Drawing for the job (mm, zero at the part's lowest x, y, z). Give positions to 0.01 mm unless a question says otherwise; leave off trailing zeros. Order: outer loops, then holes, each group sorted by start corner. A loop starts at its lowest first (then second) coordinate and runs counter-clockwise, first axis right, second up. Notation, with made-up numbers: M 24.25,-18 L 78.25,-18 A14 ccw 78.25,-14 Z; hole C 74,28.25 d2. An arc over 180 degrees is marked long. One line per item, written item: value.
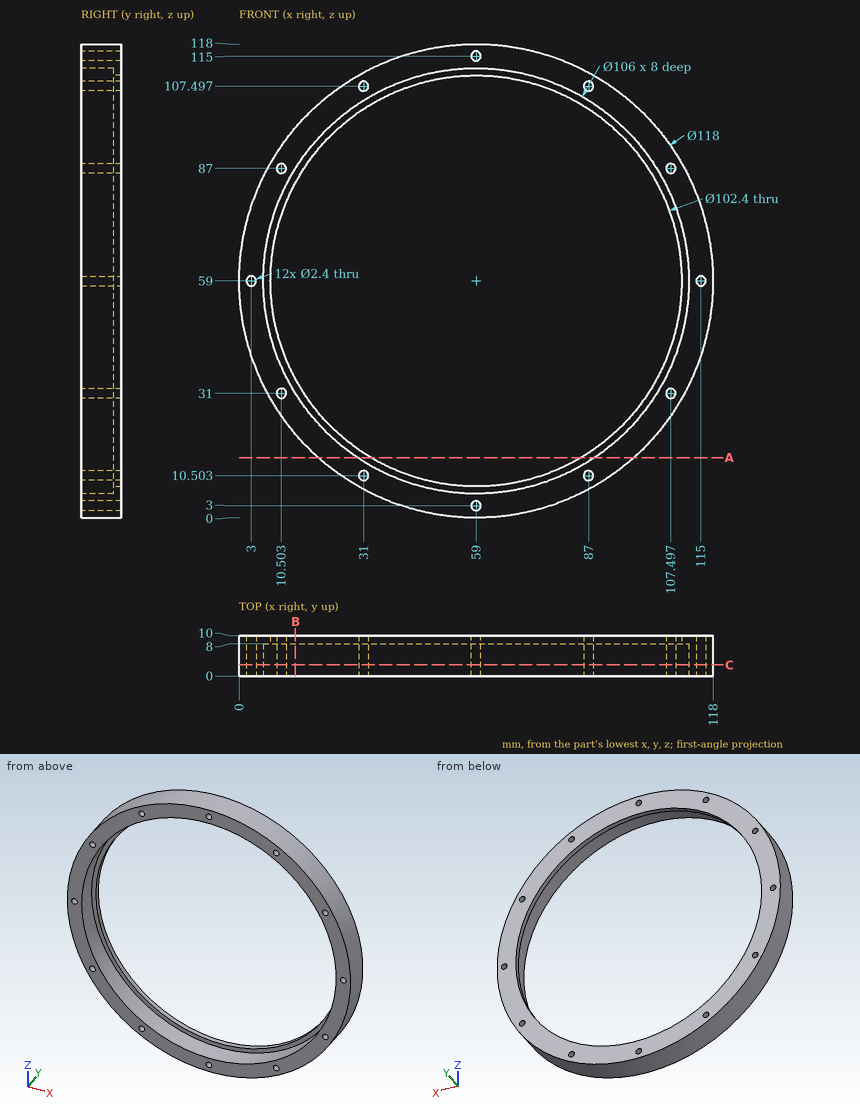
1) Saw through at C-C, the plane y = 2.75. Give the number of separate pieces and of enclosed holes in the cut face, then the cut area to 3 significant figures.
Check values:
separate pieces: 1
enclosed holes: 13
area: 2,060 mm^2
2) Pin check, flat tips, straight feed: pin 1 (1.9 mm diameter, centred on x = 107.5, z = 87, fed in from -Y); pin 2 (3 mm diameter, centred on x = 56, y = 1, fed in from +Z); pin 3 (4 mm diameter, centred on y = 3, z = 98, fed in from -X); pin 4 (1.5 mm diameter, centred on x = 91, y = 8, fed in from -Z) (1 decimal). Stop position of each tip, or through.
Check values:
pin 1: through
pin 2: z = 117.98
pin 3: x = 13.04
pin 4: z = 9
3) Drill centre lines: probe 1 along Z at (x, y) = (59, 8.4); probe 2 along Z at (x, y) = (59, 7.75); probe 3 along X at (y, z) = (1.5, 77). Where is each one in solid material? Low to high. Write a range as from..to.
Check values:
probe 1: 0..1.8, 4.2..7.8, 110.2..113.8, 116.2..118
probe 2: 0..1.8, 4.2..6, 112..113.8, 116.2..118
probe 3: 2.81..9.15, 108.85..115.19
4) Saw through at B-B, the plane x = 14. Write the cut outline in (y, z).
Check values:
outline: M 0,20.84 L 10,20.84 L 10,34.58 L 8,34.58 L 8,31 L 0,31 Z; M 0,87 L 8,87 L 8,83.42 L 10,83.42 L 10,97.16 L 0,97.16 Z
5) Saw through at A-A, the plane z = 15. Write the cut outline in (x, y).
Check values:
outline: M 19.69,0 L 29.45,0 L 29.45,8 L 32.82,8 L 32.82,10 L 19.69,10 Z; M 85.18,8 L 88.55,8 L 88.55,0 L 98.31,0 L 98.31,10 L 85.18,10 Z
